```python
from build123d import *

# Parameters (mm, degrees)
SKETCH1_R               = 30.35
SKETCH1_R_2             = 25.35
SKETCH1_R_3             = 20.35
BOSS_EXTRUDE2_DEPTH     = 375
SKETCH1_3_R             = 25.35
SKETCH1_3_R_2           = 20.35
BOSS_EXTRUDE3_DEPTH     = 40
CUT_EXTRUDE3_START      = -275
CUT_EXTRUDE3_DEPTH      = 275
SKETCH8_R               = 1.05
CUT_EXTRUDE5_DEPTH      = 137
CUT_EXTRUDE6_DEPTH      = 137
CUT_EXTRUDE6_DEPTH_BACK = 137
SKETCH9_R               = 4.05
SKETCH10_R              = 4.05
CUT_EXTRUDE7_DEPTH      = 137


with BuildPart() as part:
    # Sketch1 → Boss-Extrude2 (new body)
    # profile 1 of 3: a face of its own
    with BuildSketch(Plane(origin=(0, 0, 0), x_dir=(1, 0, 0), z_dir=(0, 1, 0))):
        with Locations(Location((0, 0, 0), (0, 0, 270))):
            Circle(SKETCH1_R)
        Circle(SKETCH1_R_2, mode=Mode.SUBTRACT)
    # profile 2 of 3: a face of its own
    with BuildSketch(Plane(origin=(0, 0, 0), x_dir=(1, 0, 0), z_dir=(0, 1, 0))):
        Circle(SKETCH1_R_2)
        Circle(SKETCH1_R_3, mode=Mode.SUBTRACT)
    # profile 3 of 3: a face of its own
    with BuildSketch(Plane(origin=(0, 0, 0), x_dir=(1, 0, 0), z_dir=(0, 1, 0))):
        Circle(SKETCH1_R_3)
    extrude(amount=BOSS_EXTRUDE2_DEPTH)

    # Sketch1_3 → Boss-Extrude3 (add)
    with BuildSketch(Plane(origin=(0, 0, 0), x_dir=(1, 0, 0), z_dir=(0, 1, 0))):
        with Locations(Location((0, 0, 0), (0, 0, 270))):
            Circle(SKETCH1_3_R)
        with Locations(Location((0, 0, 0), (0, 0, 270))):
            Circle(SKETCH1_3_R_2, mode=Mode.SUBTRACT)
    extrude(amount=-BOSS_EXTRUDE3_DEPTH)

    # Sketch6 → Cut-Extrude3 (cut)
    with BuildSketch(Plane(origin=(0, 375, 0), x_dir=(1, 0, 0), z_dir=(0, 1, 0)).offset(CUT_EXTRUDE3_START)):
        with BuildLine():
            ThreePointArc((-29.046213178, -8.8), (0, -30.35), (29.046213178, -8.8))
            Line((29.046213178, -8.8), (-29.046213178, -8.8))
        make_face()
        with BuildLine():
            Line((-29.046213178, 8.8), (29.046213178, 8.8))
            ThreePointArc((29.046213178, 8.8), (0, 30.35), (-29.046213178, 8.8))
        make_face()
    extrude(amount=CUT_EXTRUDE3_DEPTH, mode=Mode.SUBTRACT)

    # Sketch8 → Cut-Extrude5 (cut)
    with BuildSketch(Plane.XY.offset(30.35)):
        with Locations((5.215, 50)):
            Circle(SKETCH8_R)
        with Locations((-5.215, 50)):
            Circle(SKETCH8_R)
        with Locations((-5.215, 70)):
            Circle(SKETCH8_R)
        with Locations((5.215, 70)):
            Circle(SKETCH8_R)
        with Locations((-5.215, 90)):
            Circle(SKETCH8_R)
        with Locations((5.215, 90)):
            Circle(SKETCH8_R)
        with Locations((5.215, 30)):
            Circle(SKETCH8_R)
        with Locations((-5.215, 30)):
            Circle(SKETCH8_R)
        with Locations((5.215, 10)):
            Circle(SKETCH8_R)
        with Locations((-5.215, 10)):
            Circle(SKETCH8_R)
    extrude(amount=-CUT_EXTRUDE5_DEPTH, mode=Mode.SUBTRACT)

    # Sketch9 → Cut-Extrude6 (cut, two sides: drawn at the far end of the back side and taken through both)
    with BuildSketch(Plane(origin=(0, 0, 0), x_dir=(0, 0, -1), z_dir=(1, 0, 0)).offset(-CUT_EXTRUDE6_DEPTH_BACK)):
        with Locations(Location((0, -20, 0), (0, 0, 180))):
            Circle(SKETCH9_R)
    extrude(amount=CUT_EXTRUDE6_DEPTH + CUT_EXTRUDE6_DEPTH_BACK, mode=Mode.SUBTRACT)

    # Sketch10 → Cut-Extrude7 (cut)
    with BuildSketch(Plane(origin=(0, 0, -8.8), x_dir=(-1, 0, 0), z_dir=(0, 0, -1))):
        with Locations((20, 110)):
            Circle(SKETCH10_R)
        with Locations((-20, 110)):
            Circle(SKETCH10_R)
        with Locations((-20, 160)):
            Circle(SKETCH10_R)
        with Locations((20, 160)):
            Circle(SKETCH10_R)
        with Locations((-20, 210)):
            Circle(SKETCH10_R)
        with Locations((20, 210)):
            Circle(SKETCH10_R)
        with Locations((-20, 260)):
            Circle(SKETCH10_R)
        with Locations((20, 260)):
            Circle(SKETCH10_R)
        with Locations((-20, 310)):
            Circle(SKETCH10_R)
        with Locations((20, 310)):
            Circle(SKETCH10_R)
        with Locations((-20, 360)):
            Circle(SKETCH10_R)
        with Locations((20, 360)):
            Circle(SKETCH10_R)
    extrude(amount=-CUT_EXTRUDE7_DEPTH, mode=Mode.SUBTRACT)


solid = part.part
```
Here's how the part is built. I have some questions about the finished solid (model axes, mm). A direction names the side the tool comes from. Coordinates: 2 decimals unless noted, no trailing zeros. Order: outer loops, then holes, each group sorted by start corner. A loop starts at its lowest first (then second) coordinate and runs counter-clockwise, first axis right, second up.
Item 1: I need wall thicknesses on probe 1 along X at (y, z) = (360, -1.5); probe 2 along X at (y, z) = (-14, 0); probe 3 along Z at (x, y) = (13.5, 129.5). Which ranges of each line are inside material? Lowest first, please.
Response values:
probe 1: x = -30.31 to -24.05, -15.95 to 15.95, 24.05 to 30.31
probe 2: x = -25.35 to -20.35, 20.35 to 25.35
probe 3: z = -8.8 to 8.8
Item 2: If we section it at A-A, the plane y = 160: List the corners of the cut face in (x, z) for me, then the cut area to 3 significant figures.
Response values:
outline: (-29.05, -8.8) - (-24.05, -8.8) - (-24.05, 8.8) - (-29.05, 8.8) arc R30.35 ccw to start; (-15.95, -8.8) - (15.95, -8.8) - (15.95, 8.8) - (-15.95, 8.8) - close; (24.05, -8.8) - (29.05, -8.8) arc R30.35 ccw to (29.05, 8.8) - (24.05, 8.8) - close
area: 768 mm2
Item 3: Which directions (+Z, -Z, +X, -X, +Y, -Y) give clear straight access to the entire face, cutting with the end or side of a thin tool? Please do faces 1 (the face through (0, 100, -17)), 2 (the face through (0, 100, 17)), 3 (the face through (-19.866, -19.72, -4.411)), 4 (the face through (-19.122, 356.046, -0.123)).
Response values:
face 1: -Z, +X, -X, +Y
face 2: +Z, +X, -X, +Y
face 3: -Y
face 4: +Z, -Z
Item 4: I'm going to push flat-ended pins straight in: pin 1 Ø5 at (x, y) = (20, 260) entering from -Z; pin 2 Ø9.5 at (x, y) = (-20, 110) entering from -Z; pin 3 Ø4 at (x, y) = (22.5, 256) entering from +Z; pin 4 Ø12 at (y, z) = (20.5, 15) entering from +X. Where does each tip first touch, or does it pass through?
Response values:
pin 1: passes through
pin 2: stops at z = -8.8
pin 3: stops at z = 8.8
pin 4: stops at x = 28.98
Item 5: If we section it at C-C, the plane x = 10.5: List the corners of the cut face in (y, z) for me.
Response values:
outline: (-40, -23.07) - (0, -23.07) - (0, -28.48) - (100, -28.48) - (100, -8.8) - (375, -8.8) - (375, 8.8) - (100, 8.8) - (100, 28.48) - (0, 28.48) - (0, 23.07) - (-40, 23.07) - (-40, 17.43) - (0, 17.43) - (0, -17.43) - (-40, -17.43) - close
Item 6: If we section it at D-D, the plane y = 241: List the corners of the cut face in (x, z) for me.
Response values:
outline: (-29.05, -8.8) - (29.05, -8.8) arc R30.35 ccw to (29.05, 8.8) - (-29.05, 8.8) arc R30.35 ccw to start
Item 7: If we section it at B-B, the plane z = 0: Give the number of separate pieces and of enclosed holes in the cut face, then the cut area to 3 significant figures.
Response values:
separate pieces: 3
enclosed holes: 22
area: 22,400 mm2
Item 8: Thinking about a two-plate mould opening in Z: for faces 5 (the face through (-19.122, 106.046, -0.123)), 6 (the face through (0, 236, 8.8)), 7 (the face through (-24.747, -19.72, -5.495)), 8 (the face through (0, 0, 0)), which applies, pulls with the +Z half, pulls with the -Z half, needs draft (parallel to the pull), parting line crosses it, or undercut?
Response values:
face 5: needs draft
face 6: pulls with the +Z half
face 7: parting line crosses it
face 8: undercut
